Can you work these out from the model? Positions are in its coordinate system, mm. Face numbers are marked on the shaded views. A direction names the side the tool comes from. Give positions to 0.01 mm unless a question says otherwise; leave off trailing zeros.
Autodesk Inventor part; units mm, degrees
ref_plane "YZ Plane" through (0, 0, 0) normal (1, 0, 0) x (0, 1, 0)
ref_plane "XZ Plane" through (0, 0, 0) normal (0, 1, 0) x (-1, 0, 0)
ref_plane "XY Plane" through (0, 0, 0) normal (0, 0, 1) x (1, 0, 0)
sketch "Sketch1" plane through (0, 0, 0) normal (0, 1, 0) x (-1, 0, 0)
  circle A0 centre (0, 0) radius 25.4
  line L0 (-28.575, 28.575) -> (28.575, 28.575)
  line L1 (28.575, 28.575) -> (28.575, -28.575)
  line L2 (28.575, -28.575) -> (-28.575, -28.575)
  line L3 (-28.575, -28.575) -> (-28.575, 28.575)
  line L4 (-28.575, 28.575) -> (28.575, -28.575) construction
  line L5 (28.575, 28.575) -> (-28.575, -28.575) construction
  line L6 (-26.9875, 26.9875) -> (26.9875, 26.9875)
  line L7 (26.9875, 26.9875) -> (26.9875, -26.9875)
  line L8 (26.9875, -26.9875) -> (-26.9875, -26.9875)
  line L9 (-26.9875, -26.9875) -> (-26.9875, 26.9875)
  line L10 (-26.9875, 26.9875) -> (26.9875, -26.9875) construction
  line L11 (26.9875, 26.9875) -> (-26.9875, -26.9875) construction
  dimension "d0" = 50.8
  dimension "d2" = 28.575
  dimension "d7" = 26.9875
extrude "Extrusion1" add sketch "Sketch1" against normal blind 8.509 contours L0 L1 L2 L3
extrude "Extrusion2" add sketch "Sketch1" along normal blind 1.27 contours L0 L1 L2 L3 | L6 L7 L8 L9
fillet "Fillet1" radius 3.175 4 edges at (-28.575, -3.6195, -28.575) (28.575, -3.6195, -28.575) (28.575, -3.6195, 28.575) (-28.575, -3.6195, 28.575)
fillet "Fillet2" radius 3.175 8 edges at (27.6451, 1.27, -27.6451) (0, 1.27, -28.575) (-27.6451, 1.27, -27.6451) (-28.575, 1.27, 0) (-27.6451, 1.27, 27.6451) (0, 1.27, 28.575) (27.6451, 1.27, 27.6451) (28.575, 1.27, 0)
properties part number "TrackDisplayTop"
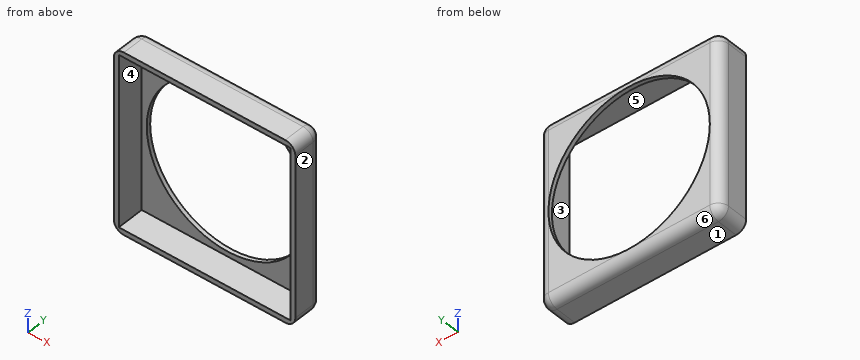
1) For the marked faces 5 and 6, which set-ups out of +Z, -Z, +X, -X, +Y, -Y let a thin tool reach every point of the face, with its end or its side?
Values follow:
face 5: -Y
face 6: -Z, +X, -X, +Y
2) For pin 1 Ø2 at (x, z) = (22.5, -20.5) entering from -Y, with a flat end and sliding along its axis, tell me the tip position at first contact or that it passes through.
Values follow:
pin 1: stops at y = 0
3) If we mould it in two halves opening along Z, with no side actions, what happens to the marked faces 1, 2, 3 and 4? For each: +Z half, -Z half, draft (parallel to the pull), parting line (faces both ways), or undercut.
Values follow:
face 1: -Z half
face 2: draft
face 3: undercut
face 4: undercut
4) Please list where these lines run through material, in increasing order: L1, parallel to X at y = -5.5, z = 3 (1 decimal); L2, parallel to Z at x = 0, y = 0.5.
Values follow:
L1: x = -28.6 to -27, 27 to 28.6
L2: z = -27.47 to -25.4, 25.4 to 27.47
